Verification items for the finished model (mm, model axes). Face numbers are marked on the shaded views. Round coordinates to 2 decimals unless told otherwise and drop trailing zeros. Order: outer loops, then holes, each group sorted by start corner. A loop starts at its lowest first (then second) coordinate and runs counter-clockwise, first axis right, second up. Notation, with made-up numbers: M 8,74.5 L 61,74.5 A29 ccw 61,106.5 Z; hole C 21.5,-27.5 d1. An arc over 180 degrees is marked long. Return JSON: item names as keys, results as strings. Group by question number.
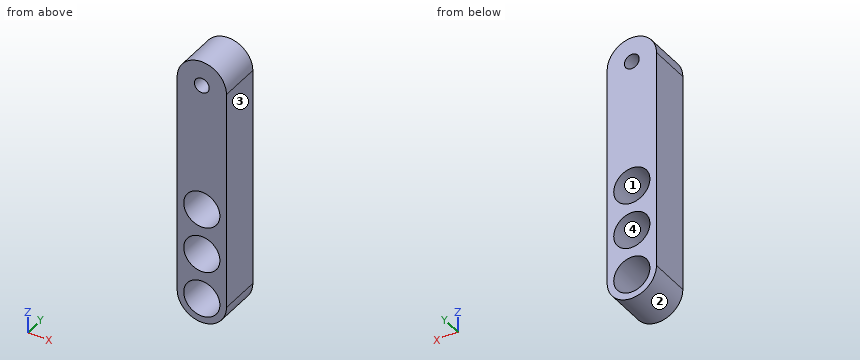
from build123d import *

# Parameters (mm, degrees)
SKETCH1_R           = 1.125
SKETCH1_R_2         = 2.75
BOSS_EXTRUDE1_DEPTH = 6.35
SKETCH2_R           = 2.75
CUT_EXTRUDE2_DEPTH  = 6.35


with BuildPart() as part:
    # Sketch1 → Boss-Extrude1 (new body)
    with BuildSketch(Plane(origin=(0, 0, 0), x_dir=(1, 0, 0), z_dir=(0, 1, 0))):
        with BuildLine():
            Line((-3.75, 33.5), (-3.75, 0))
            ThreePointArc((-3.75, 0), (0, -3.75), (3.75, 0))
            Line((3.75, 0), (3.75, 33.5))
            ThreePointArc((3.75, 33.5), (0, 37.25), (-3.75, 33.5))
        make_face()
        Circle(SKETCH1_R, mode=Mode.SUBTRACT)
        with Locations((0, 33.5)):
            Circle(SKETCH1_R_2, mode=Mode.SUBTRACT)
    extrude(amount=BOSS_EXTRUDE1_DEPTH)

    # Sketch2 → Cut-Extrude2 (cut)
    with BuildSketch(Plane(origin=(0, 0, 0), x_dir=(1, 0, 0), z_dir=(0, 1, 0))):
        with Locations((0, 33.5)):
            Circle(SKETCH2_R)
        with Locations((0, 19.5)):
            Circle(SKETCH2_R)
        with Locations((0, 26.5)):
            Circle(SKETCH2_R)
    extrude(amount=CUT_EXTRUDE2_DEPTH, mode=Mode.SUBTRACT)


solid = part.part
1. Cross-section at B-B (y = 5.25). Enter the section's corners in (x, z) (3 decimals), plus the area to 3 significant figures.
2. Draft check along Z on the marked faces 1, 2, 3 and 4. Enter one of: +Z half, -Z half, draft (parallel to the pull), parting line (faces both ways), or undercut.
3. Cross-section at D-D (x = 2.25). Enter the section's corners in (y, z).
4. Cross-section at C-C (z = -26.5). Enter the section's corners in (x, y), plus the area to 3 significant figures.
5. Cross-section at A-A (x = 0). Enter the section's corners in (y, z) (3 decimals), plus the area to 3 significant figures.
6. Thickness scan on line 1 along Z through (x, y) = (0, 2) (3 decimals); line 2 along X through (y, z) = (5, -19.5); line 3 along Z through (x, y) = (-2.5, 5.75). Record the ranges inside material, lowest first. Write a range as from..to.
7. Go/stop test with a flat-tipped pin: pin 1 (2 mm diameter, centred on x = 1.5, y = 2.5, fed in from -Z). Record where the tip stops, or that it passes through.
Computed:
{
 "1": {"outline": "M -3.75,-33.5 A3.75 ccw 3.75,-33.5 L 3.75,0 A3.75 ccw -3.75,0 Z; hole C 0,-33.5 d5.5; hole C 0,-26.5 d5.5; hole C 0,-19.5 d5.5; hole C 0,0 d2.25", "area": "220 mm²"},
 "2": {"face 1": "undercut", "face 2": "-Z half", "face 3": "draft", "face 4": "undercut"},
 "3": {"outline": "M 0,-36.5 L 6.35,-36.5 L 6.35,-35.08 L 0,-35.08 Z; M 0,-31.92 L 6.35,-31.92 L 6.35,-28.08 L 0,-28.08 Z; M 0,-24.92 L 6.35,-24.92 L 6.35,-21.08 L 0,-21.08 Z; M 0,-17.92 L 6.35,-17.92 L 6.35,3 L 0,3 Z"},
 "4": {"outline": "M -3.75,0 L -2.75,0 L -2.75,6.35 L -3.75,6.35 Z; M 2.75,0 L 3.75,0 L 3.75,6.35 L 2.75,6.35 Z", "area": "12.7 mm²"},
 "5": {"outline": "M 0,-37.25 L 6.35,-37.25 L 6.35,-36.25 L 0,-36.25 Z; M 0,-30.75 L 6.35,-30.75 L 6.35,-29.25 L 0,-29.25 Z; M 0,-23.75 L 6.35,-23.75 L 6.35,-22.25 L 0,-22.25 Z; M 0,-16.75 L 6.35,-16.75 L 6.35,-1.125 L 0,-1.125 Z; M 0,1.125 L 6.35,1.125 L 6.35,3.75 L 0,3.75 Z", "area": "141 mm²"},
 "6": {"line 1": "z = -37.25..-36.25, -30.75..-29.25, -23.75..-22.25, -16.75..-1.125, 1.125..3.75", "line 2": "x = -3.75..-2.75, 2.75..3.75", "line 3": "z = -36.3..-34.65, -32.35..-27.65, -25.35..-20.65, -18.35..2.8"},
 "7": {"pin 1": "stops at z = -37.22"}
}
